```python
from build123d import *

# Parameters (mm, degrees)
BOSS_EXTRU_1_DEPTH = 800


with BuildPart() as part:
    # Balayage1: sweep along a path in Esquisse1
    with BuildLine(Plane.XY) as balayage1_path:
        Line((-600, -400), (600, -400))
        Line((600, -400), (600, 400))
        Line((600, 400), (-600, 400))
        Line((-600, 400), (-600, -400))
    # Esquisse2 → Balayage1 (sweep)
    with BuildSketch(Plane(origin=(0, 0, 0), x_dir=(1, 0, 0), z_dir=(0, 1, 0))):
        with BuildLine():
            Line((-512, -15), (-488, -15))
            ThreePointArc((-488, -15), (-485.878679656, -14.121320344), (-485, -12))
            Line((-485, -12), (-485, 12))
            ThreePointArc((-485, 12), (-485.878679656, 14.121320344), (-488, 15))
            Line((-488, 15), (-512, 15))
            ThreePointArc((-512, 15), (-514.121320344, 14.121320344), (-515, 12))
            Line((-515, 12), (-515, -12))
            ThreePointArc((-515, -12), (-514.121320344, -14.121320344), (-512, -15))
        make_face()
        with BuildLine():
            Line((-510, -13), (-490, -13))
            ThreePointArc((-490, -13), (-487.878679656, -12.121320344), (-487, -10))
            Line((-487, -10), (-487, 10))
            ThreePointArc((-487, 10), (-487.878679656, 12.121320344), (-490, 13))
            Line((-490, 13), (-510, 13))
            ThreePointArc((-510, 13), (-512.121320344, 12.121320344), (-513, 10))
            Line((-513, 10), (-513, -10))
            ThreePointArc((-513, -10), (-512.121320344, -12.121320344), (-510, -13))
        make_face(mode=Mode.SUBTRACT)
    sweep(path=balayage1_path.line, transition=Transition.RIGHT)

    # Esquisse3 → Boss.-Extru.1 (add)
    # profile 1 of 4: a face of its own
    with BuildSketch(Plane.XY.offset(15)):
        with BuildLine():
            Line((-512, 285), (-488, 285))
            ThreePointArc((-488, 285), (-485.878679656, 285.878679656), (-485, 288))
            Line((-485, 288), (-485, 312))
            ThreePointArc((-485, 312), (-485.878679656, 314.121320344), (-488, 315))
            Line((-488, 315), (-512, 315))
            ThreePointArc((-512, 315), (-514.121320344, 314.121320344), (-515, 312))
            Line((-515, 312), (-515, 288))
            ThreePointArc((-515, 288), (-514.121320344, 285.878679656), (-512, 285))
        make_face()
        with BuildLine():
            Line((-510, 287), (-490, 287))
            ThreePointArc((-490, 287), (-487.878679656, 287.878679656), (-487, 290))
            Line((-487, 290), (-487, 310))
            ThreePointArc((-487, 310), (-487.878679656, 312.121320344), (-490, 313))
            Line((-490, 313), (-510, 313))
            ThreePointArc((-510, 313), (-512.121320344, 312.121320344), (-513, 310))
            Line((-513, 310), (-513, 290))
            ThreePointArc((-513, 290), (-512.121320344, 287.878679656), (-510, 287))
        make_face(mode=Mode.SUBTRACT)
    # profile 2 of 4: a face of its own
    with BuildSketch(Plane.XY.offset(15)):
        with BuildLine():
            Line((485, 288), (485, 312))
            ThreePointArc((485, 312), (485.878679656, 314.121320344), (488, 315))
            Line((488, 315), (512, 315))
            ThreePointArc((512, 315), (514.121320344, 314.121320344), (515, 312))
            Line((515, 312), (515, 288))
            ThreePointArc((515, 288), (514.121320344, 285.878679656), (512, 285))
            Line((512, 285), (488, 285))
            ThreePointArc((488, 285), (485.878679656, 285.878679656), (485, 288))
        make_face()
        with BuildLine():
            Line((487, 290), (487, 310))
            ThreePointArc((487, 310), (487.878679656, 312.121320344), (490, 313))
            Line((490, 313), (510, 313))
            ThreePointArc((510, 313), (512.121320344, 312.121320344), (513, 310))
            Line((513, 310), (513, 290))
            ThreePointArc((513, 290), (512.121320344, 287.878679656), (510, 287))
            Line((510, 287), (490, 287))
            ThreePointArc((490, 287), (487.878679656, 287.878679656), (487, 290))
        make_face(mode=Mode.SUBTRACT)
    # profile 3 of 4: a face of its own
    with BuildSketch(Plane.XY.offset(15)):
        with BuildLine():
            Line((-512, -315), (-488, -315))
            ThreePointArc((-488, -315), (-485.878679656, -314.121320344), (-485, -312))
            Line((-485, -312), (-485, -288))
            ThreePointArc((-485, -288), (-485.878679656, -285.878679656), (-488, -285))
            Line((-488, -285), (-512, -285))
            ThreePointArc((-512, -285), (-514.121320344, -285.878679656), (-515, -288))
            Line((-515, -288), (-515, -312))
            ThreePointArc((-515, -312), (-514.121320344, -314.121320344), (-512, -315))
        make_face()
        with BuildLine():
            Line((-510, -287), (-490, -287))
            ThreePointArc((-490, -287), (-487.878679656, -287.878679656), (-487, -290))
            Line((-487, -290), (-487, -310))
            ThreePointArc((-487, -310), (-487.878679656, -312.121320344), (-490, -313))
            Line((-490, -313), (-510, -313))
            ThreePointArc((-510, -313), (-512.121320344, -312.121320344), (-513, -310))
            Line((-513, -310), (-513, -290))
            ThreePointArc((-513, -290), (-512.121320344, -287.878679656), (-510, -287))
        make_face(mode=Mode.SUBTRACT)
    # profile 4 of 4: a face of its own
    with BuildSketch(Plane.XY.offset(15)):
        with BuildLine():
            Line((512, -285), (488, -285))
            ThreePointArc((488, -285), (485.878679656, -285.878679656), (485, -288))
            Line((485, -288), (485, -312))
            ThreePointArc((485, -312), (485.878679656, -314.121320344), (488, -315))
            Line((488, -315), (512, -315))
            ThreePointArc((512, -315), (514.121320344, -314.121320344), (515, -312))
            Line((515, -312), (515, -288))
            ThreePointArc((515, -288), (514.121320344, -285.878679656), (512, -285))
        make_face()
        with BuildLine():
            Line((510, -287), (490, -287))
            ThreePointArc((490, -287), (487.878679656, -287.878679656), (487, -290))
            Line((487, -290), (487, -310))
            ThreePointArc((487, -310), (487.878679656, -312.121320344), (490, -313))
            Line((490, -313), (510, -313))
            ThreePointArc((510, -313), (512.121320344, -312.121320344), (513, -310))
            Line((513, -310), (513, -290))
            ThreePointArc((513, -290), (512.121320344, -287.878679656), (510, -287))
        make_face(mode=Mode.SUBTRACT)
    extrude(amount=BOSS_EXTRU_1_DEPTH)


solid = part.part
```
Check sheet for the modelled part. Datum: model origin and axes. Units: mm. A direction names the side the tool comes from. Round coordinates to 2 decimals unless told otherwise and drop trailing zeros. Write item = value, one per line. Start each with the question number.
Q1. Depth check by flat-ended pin: P1, Ø12.5, axis at x = 496, y = -299.5, coming from the +Z side. Enter the tip coordinate at first touch or a pass-through.
Q2. Section check A-A (y = -17.5). Count the separate pieces of the cut face and the enclosed holes in it, plus the area to 3 significant figures.
Q3. Release check for a two-part mould opening along X. For faces 1 (the face through (500, -315, 409)), 2 (the face through (515, 4, 0)), 3 (the face through (485, -300, 409)) record: pulls with the +X half, pulls with the -X half, needs draft (parallel to the pull), parting line crosses it, or undercut.
Q4. Access from +Z, -Z, +X, -X, +Y, -Y to the whole of each face (thin tool, end or side, straight path). Record for faces 4 (the face through (153, 297, -13)), 5 (the face through (7, 300, 15)), 6 (the face through (485, 4, 0)).
Derived:
q1.P1 = 15
q2.separate_pieces = 2
q2.enclosed_holes = 2
q2.area = 448 mm^2
q3.face_1 = needs draft
q3.face_2 = pulls with the +X half
q3.face_3 = undercut
q4.face_4 = none
q4.face_5 = +Z, +Y, -Y
q4.face_6 = +Z, -Z
